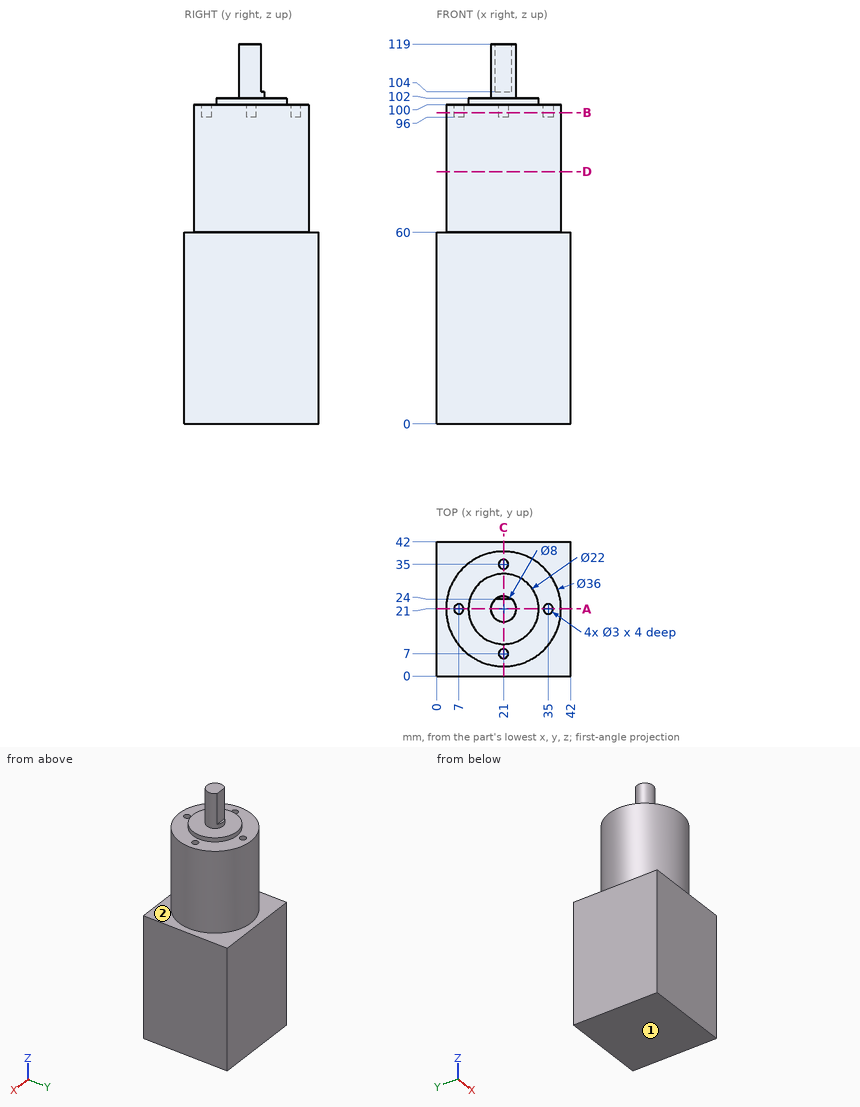
Design review of the part shown in the three views and the two pictorial views. Dimensions are in mm from the part's minimum x, y and z. A direction names the side the tool comes from. Round coordinates to 2 decimals unless told otherwise and drop trailing zeros. Loops run counter-clockwise (first coordinate to the right, second up) from the corner with the lowest first, then second, coordinate; pieces in that order, holes last. Notation, with made-up numbers: (52, 83) -> (90, 83) arc R15 ccw to (90, 92) -> close; hole circle Ø7 at (-5, 33.25). An arc over 180 degrees is marked (long way). Answer as a JSON object with one key per item and string values. Group by question number.
1) We need section A-A on y = 21. Write out the cut boundary in (x, z), then the cut area to 3 significant figures.
2) For line 1 (Y direction, x = 21, z = 98.3); line 2 (Z direction, x = 17, y = 17); line 3 (Z direction, x = 4, y = 2), list the stretches that pass through material, from the lowest coordinate up. Write a range as [from, to].
3) For the marked faces 1 and 2, list the 3-axis set-ups (+Z, -Z, +X, -X, +Y, -Y) from which the entire face can be reached by the end or side of a thin tool; tool diameter is ignored.
4) We need section D-D on z = 79. Write out the cut boundary in (x, y).
5) We need section B-B on z = 97.5. Write out the cut boundary in (x, y).
6) For pin 1 Ø5 at (x, y) = (21, 7) entering from +Z; pin 2 Ø1 at (x, y) = (11.5, 21.5) entering from +Z; pin 3 Ø4 at (x, z) = (20, 109) entering from +Y, all flat-tipped, find the tip position at first contact; note any pin that passes through.
7) We need section C-C on x = 21. Write out the cut boundary in (y, z).
Result set:
{
 "1": {"outline": "(0, 0) -> (42, 0) -> (42, 60) -> (39, 60) -> (39, 100) -> (36.5, 100) -> (36.5, 96) -> (33.5, 96) -> (33.5, 100) -> (32, 100) -> (32, 102) -> (25, 102) -> (25, 119) -> (17, 119) -> (17, 102) -> (10, 102) -> (10, 100) -> (8.5, 100) -> (8.5, 96) -> (5.5, 96) -> (5.5, 100) -> (3, 100) -> (3, 60) -> (0, 60) -> close", "area": "4,120 mm²"},
 "2": {"line 1": "[3, 5.5], [8.5, 33.5], [36.5, 39]", "line 2": "[0, 102]", "line 3": "[0, 60]"},
 "3": {"face 1": "-Z, +X, -X, +Y, -Y", "face 2": "+Z"},
 "4": {"outline": "circle Ø36 at (21, 21)"},
 "5": {"outline": "circle Ø36 at (21, 21); hole circle Ø3 at (7, 21); hole circle Ø3 at (21, 7); hole circle Ø3 at (21, 35); hole circle Ø3 at (35, 21)"},
 "6": {"pin 1": "z = 100", "pin 2": "z = 102", "pin 3": "y = 24"},
 "7": {"outline": "(0, 0) -> (42, 0) -> (42, 60) -> (39, 60) -> (39, 100) -> (36.5, 100) -> (36.5, 96) -> (33.5, 96) -> (33.5, 100) -> (32, 100) -> (32, 102) -> (25, 102) -> (25, 104) -> (24, 104) -> (24, 119) -> (17, 119) -> (17, 102) -> (10, 102) -> (10, 100) -> (8.5, 100) -> (8.5, 96) -> (5.5, 96) -> (5.5, 100) -> (3, 100) -> (3, 60) -> (0, 60) -> close"}
}
